Part model, mm, in its own coordinate system. A direction names the side the tool comes from. Coordinates: 2 decimals unless noted, no trailing zeros. Loops run counter-clockwise (first coordinate to the right, second up) from the corner with the lowest first, then second, coordinate; pieces in that order, holes last. Notation, with made-up numbers: (-8, -9) - (45, -9) arc R26 ccw to (45, 8) - close; hole circle Ø2 at (59, 2.25). An arc over 180 degrees is marked (long way). Use a Markdown table: item, result. Add a question column.
1. 3-axis set-ups, long thin cutter, end or side, ignore diameter. For faces 4 (the cylindrical face through (-1.587, 12.088, 2.576)), 5 (the conical face through (-2.17, -9.75, 16.39)), 6 (the flat face through (0, 0, 0)), 7 (the cylindrical face through (-1.587, 12.088, 53.78)): which of +Z, -Z, +X, -X, +Y, -Y reach the whole face in a straight line?
2. Pull direction Z, two halves, no side cores. Call faces 1 (the cylindrical face through (0.83, -3.72, 36.67)), 2 (the flat face through (0.1, 12.5, 10.16)), 3 (the conical face through (9.256, -3.838, 49.232)): pulls with the +Z half, pulls with the -Z half, needs draft (parallel to the pull), parting line crosses it, or undercut.
3. Band-saw the part on A-A, the plane z = 34. Give the cut face in (x, y), plus the area to 3 significant figures.
4. Band-saw the part on B-B, the plane z = 15. Give the cut face in (x, y).
5. Wall check: probe 1 along Y at (x, z) = (0, 37); probe 2 along Y at (x, z) = (0, 51.9). Give the ranges that are in metal, low to high. Write a range as [from, to].
6. Drop flat-ended pins along their axis: pin 1 (10 mm diameter, centred on y = -8.5, z = 46, fed in from -X); pin 2 (4.5 mm diameter, centred on x = 0, y = 0, fed in from +Z); pin 3 (15 mm diameter, centred on x = -7, y = 4, fed in from +Z); pin 4 (3 mm diameter, centred on x = -4, z = 39.5, fed in from -Y). Give the stop position or say it passes through.
from build123d import *

# Parameters (mm, degrees)
F0_W         = 6.096
F0_H         = 5.08
F0_W_2       = 3.048
F0_H_2       = 5.2907199979
F0_W_3       = 6.604
F2_SIZE      = 2.54
F3_SIZE      = 2.54
F5_D         = 7.62
F5_DEPTH     = 25.4
F5_TIP       = 2.2892789585
F6_W         = 7.272795774
F6_H         = 32.1356244385
F8_S5_R      = 9.8747471347
F8_T6_DEPTH  = 19
F8_S11_R     = 9.8747471347
F8_T12_DEPTH = 19


# Not quite as in the source:
# - a fillet or chamfer that OpenCascade refuses, or shapes differently, is made with other operations: its cross-section is extruded or revolved along the edge and cut away or added


with BuildPart() as f1:
    # F0 (on Front) → F1 (revolve)
    with BuildSketch(Plane.XZ):
        with Locations((9.144, 2.54)):
            Rectangle(F0_W, F0_H)
        Polygon((0, 50.8), (0, 47.4797748029), (6.096, 50.8), align=None)
        with Locations((9.144, 7.62)):
            Rectangle(F0_W, F0_H)
        with Locations((10.668, 53.4453599989)):
            Rectangle(F0_W_2, F0_H_2)
        Polygon((0, 47.4797748029), (0, 0), (6.096, 0), (6.096, 5.08), (6.096, 10.16), (12.192, 10.16), (12.192, 50.8), (9.144, 50.8), (6.096, 50.8), align=None)
        with Locations((15.494, 7.62)):
            Rectangle(F0_W_3, F0_H)
    revolve(axis=Axis((0, 0, 25.4), (0, 0, 1)))

    # F2
    f2_edges = [f1.edges().sort_by_distance(p)[0] for p in [
        (-9.144, 0, 56.09072),
    ]]
    chamfer(f2_edges, length=F2_SIZE)

    # F3
    f3_edges = [f1.edges().sort_by_distance(p)[0] for p in [
        (-18.796, 0, 10.16),
    ]]
    chamfer(f3_edges, length=F3_SIZE)

    # F5
    with Locations(Plane.XY.offset(50.8)):
        with Locations((0, 0)):
            Hole(F5_D / 2, depth=F5_DEPTH)
            with Locations((0, 0, -(F5_DEPTH + F5_TIP / 2))):  # 118° drill point
                Cone(0, F5_D / 2, F5_TIP, mode=Mode.SUBTRACT)

    # F6 (on Right) → F7 (revolve, cut)
    with BuildSketch(Plane.YZ):
        with Locations((-13.5111450218, 32.7963028103)):
            Rectangle(F6_W, F6_H)
    revolve(axis=Axis((0, 0, 32.7963028103), (0, 0, -1)), mode=Mode.SUBTRACT)

    # F8: chamfer of 2.54 on 5 edges, made by hand


with BuildPart() as f8_tool2:
    # F8_s3 → F8_t4 (revolve)
    with BuildSketch(Plane.XZ):
        Polygon((9.652, 48.8641150296), (12.192, 51.4041150296), (12.192, 48.8641150296), align=None)
    revolve(axis=Axis((0, 0, 48.8641150296), (0, 0, 1)))

    # F8_s5 → F8_t6 (cut, symmetric)
    with BuildSketch(Plane.XY.offset(50.1)):
        Circle(F8_S5_R)
    extrude(amount=F8_T6_DEPTH, both=True, mode=Mode.SUBTRACT)


with BuildPart() as f1_1:
    add(f1.part)

    # F8_t1: cut F8_tool2
    add(f8_tool2.part, mode=Mode.SUBTRACT)


with BuildPart() as f8_tool8:
    # F8_s9 → F8_t10 (revolve)
    with BuildSketch(Plane.XZ):
        Polygon((12.192, 14.188490591), (9.652, 16.728490591), (12.192, 16.728490591), align=None)
    revolve(axis=Axis((0, 0, 16.728490591), (0, 0, 1)))

    # F8_s11 → F8_t12 (cut, symmetric)
    with BuildSketch(Plane.XY.offset(15.5)):
        Circle(F8_S11_R)
    extrude(amount=F8_T12_DEPTH, both=True, mode=Mode.SUBTRACT)


with BuildPart() as f1_2:
    add(f1_1.part)

    # F8_t7: cut F8_tool8
    add(f8_tool8.part, mode=Mode.SUBTRACT)

    # F8_s13 → F8_t14 (revolve, cut)
    with BuildSketch(Plane.XZ):
        Polygon((15.2038975516, 10.16), (16.9999487758, 9.4160512242), (16.256, 10.16), align=None)
    revolve(axis=Axis((0, 0, 10.16), (0, 0, 1)), mode=Mode.SUBTRACT)

    # F8_s15 → F8_t16 (revolve, cut)
    with BuildSketch(Plane.XZ):
        Polygon((18.0520512242, 8.3639487758), (18.796, 6.5678975516), (18.796, 7.62), align=None)
    revolve(axis=Axis((0, 0, 7.62), (0, 0, 1)), mode=Mode.SUBTRACT)

    # F8_s17 → F8_t18 (revolve, cut)
    with BuildSketch(Plane.XZ):
        Polygon((6.35, 50.8), (3.81, 48.26), (3.81, 50.8), align=None)
    revolve(axis=Axis((0, 0, 50.8), (0, 0, 1)), mode=Mode.SUBTRACT)


solid = f1_2.part
Geometry check:
| question | item | result |
|---|---|---|
| 1 | face 4 | -Z |
| 1 | face 5 | none |
| 1 | face 6 | -Z, +X, -X, +Y, -Y |
| 1 | face 7 | +Z |
| 2 | face 1 | needs draft |
| 2 | face 2 | pulls with the +Z half |
| 2 | face 3 | undercut |
| 3 | outline | circle Ø19.75 at (0, 0); hole circle Ø7.62 at (0, 0) |
| 3 | area | 261 mm^2 |
| 4 | outline | circle Ø22.76 at (0, 0) |
| 5 | probe 1 | y = [-9.87, -3.81], [3.81, 9.87] |
| 5 | probe 2 | y = [-12.19, -9.14], [9.14, 12.19] |
| 6 | pin 1 | stops at x = -9.36 |
| 6 | pin 2 | stops at z = 24.46 |
| 6 | pin 3 | stops at z = 56.09 |
| 6 | pin 4 | stops at y = -9.55 |
